Here's how the part is built. I have some questions about the finished solid (model axes, mm). A direction names the side the tool comes from. Give positions to 0.01 mm unless a question says otherwise; leave off trailing zeros. Order: outer loops, then holes, each group sorted by start corner. A loop starts at its lowest first (then second) coordinate and runs counter-clockwise, first axis right, second up. Notation, with made-up numbers: (20.5, -31) - (56.5, -31) arc R17 cw to (56.5, -19) - close; hole circle Ø7 at (51.5, 43). An arc over 180 degrees is marked (long way). One line per question, with ' | ' between items.
from build123d import *

# Parameters (mm, degrees)
SKETCH2_R      = 3.96875
SKETCH3_R      = 7.14375
EXTRUDE1_DEPTH = 5.55625
SKETCH4_R      = 3.96875
EXTRUDE2_DEPTH = 9.525
FILLET1_R      = 1.27


with BuildPart() as part:
    # Sweep1: sweep along a path in Sketch1
    with BuildLine(Plane(origin=(0, 0, 0), x_dir=(1, 0, 0), z_dir=(0, 1, 0))) as sweep1_path:
        Line((0, 0), (0, 45.72))
        ThreePointArc((0, 45.72), (1.487897552, 49.312102448), (5.08, 50.8))
        Line((5.08, 50.8), (96.52, 50.8))
        ThreePointArc((96.52, 50.8), (100.112102448, 49.312102448), (101.6, 45.72))
        Line((101.6, 45.72), (101.6, 0))
    # Sketch2 → Sweep1 (sweep)
    with BuildSketch(Plane.XY):
        Circle(SKETCH2_R)
    sweep(path=sweep1_path.line)

    # Sketch3 → Extrude1 (add, symmetric)
    with BuildSketch(Plane(origin=(0, 0, 0), x_dir=(1, 0, 0), z_dir=(0, 1, 0))):
        with Locations(Location((0, 0, 0), (0, 0, 270))):
            Circle(SKETCH3_R)
        with Locations(Location((101.6, 0, 0), (0, 0, 270))):
            Circle(SKETCH3_R)
    extrude(amount=EXTRUDE1_DEPTH, both=True)

    # Sketch4 → Extrude2 (add)
    with BuildSketch(Plane.XZ.offset(5.55625)):
        with Locations(Location((0, 0, 0), (0, 0, 90))):
            Circle(SKETCH4_R)
        with Locations(Location((101.6, 0, 0), (0, 0, 90))):
            Circle(SKETCH4_R)
    extrude(amount=EXTRUDE2_DEPTH)

    # Fillet1
    fillet1_edges = [part.edges().sort_by_distance(p)[0] for p in [
        (0, 5.55625, -7.14375),
        (101.6, 5.55625, -7.14375),
    ]]
    fillet(fillet1_edges, radius=FILLET1_R)


solid = part.part
1) I want a section at A-A (z = 0). List the corners of the cut face in (x, y) for me, plus the area to 3 significant figures.
Model answer:
outline: (-7.14, -5.56) - (-3.97, -5.56) - (-3.97, -15.08) - (3.97, -15.08) - (3.97, -5.56) - (7.14, -5.56) - (7.14, 4.29) arc R1.27 ccw to (5.87, 5.56) - (-5.87, 5.56) arc R1.27 ccw to (-7.14, 4.29) - close; (94.46, -5.56) - (97.63, -5.56) - (97.63, -15.08) - (105.57, -15.08) - (105.57, -5.56) - (108.74, -5.56) - (108.74, 4.29) arc R1.27 ccw to (107.47, 5.56) - (95.73, 5.56) arc R1.27 ccw to (94.46, 4.29) - close | area: 467 mm2
2) I want a section at C-C (y = 0). List the corners of the cut face in (x, z) for me, plus the area to 3 significant figures.
Model answer:
outline: (-3.97, -45.72) arc R9.05 ccw to (5.08, -54.77) - (96.52, -54.77) arc R9.05 ccw to (105.57, -45.72) - (105.57, -5.94) arc R7.14 ccw (long way) to (97.63, -5.94) - (97.63, -45.72) arc R1.11 cw to (96.52, -46.83) - (5.08, -46.83) arc R1.11 cw to (3.97, -45.72) - (3.97, -5.94) arc R7.14 ccw (long way) to (-3.97, -5.94) - close | area: 1,790 mm2
3) Thinking about a two-plate mould opening in Z: for faces 1 (the face through (102, 5.556, 0)), 2 (the face through (-2.736, -0.704, 6.599)), 3 (the face through (105.474, -10.252, -0.86)), which applies, +Z half, -Z half, draft (parallel to the pull), parting line (faces both ways), or undercut?
Model answer:
face 1: draft | face 2: undercut | face 3: parting line
4) I'm going to push flat-ended pins straight in: P1, Ø4, axis at y = -6.5, z = -6, coming from the +X side; P2, Ø8, axis at x = 5.5, z = -40.5, coming from the -Y side; P3, Ø6, axis at y = -2.5, z = -45, coming from the -X side. Where does each tip first touch, or does it pass through?
Model answer:
P1: stops at x = 107.35 | P2: stops at y = -3.67 | P3: stops at x = -3.97
5) I want a section at B-B (y = -10.75). List the corners of the cut face in (x, z) for me.
Model answer:
outline: circle Ø7.94 at (0, 0); circle Ø7.94 at (101.6, 0)
6) Please list where these lines run through material, in increasing order: L1, parallel to X at y = -3.75, z = 0; L2, parallel to X at y = -5.75, z = 0; L3, parallel to Z at x = 28, y = -1.5.
Model answer:
L1: x = -7.14 to 7.14, 94.46 to 108.74 | L2: x = -3.97 to 3.97, 97.63 to 105.57 | L3: z = -54.47 to -47.13
7) On a 3-axis mill with a long thin cutter (end or side, diameter ignored), from which of +Z, -Z, +X, -X, +Y, -Y can I reach the whole of each face in a straight line? I mean faces 4 (the face through (51.44, 2.415, -53.949)), 5 (the face through (0, -15.081, 0)), 6 (the face through (-3, -5.556, 3)). Say none if no direction works.
Model answer:
face 4: none | face 5: +Z, -Z, +X, -X, -Y | face 6: -Y
